```python
from build123d import *

# Parameters (mm, degrees)
ESTRUSIONE_ESTRUSIONE1_DEPTH = 4.1
SCHIZZO2_R                   = 1.25
TAGLIO_ESTRUSIONE1_DEPTH     = 4.1
RACCORDO1_DEPTH              = 4.1
RACCORDO2_R                  = 11


with BuildPart() as part:
    # Schizzo1 → Estrusione-Estrusione1 (new body)
    with BuildSketch(Plane.XY):
        with BuildLine():
            Line((-12, 0), (-12, 8))
            Line((-12, 8), (23.997894166, 8))
            Line((23.997894166, 8), (38.008621711, 8))
            Line((38.008621711, 8), (38.008621711, -12))
            Line((38.008621711, -12), (0, -12))
            ThreePointArc((0, -12), (-8.485281374, -8.485281374), (-12, 0))
        make_face()
    extrude(amount=ESTRUSIONE_ESTRUSIONE1_DEPTH)

    # Schizzo2 → Taglio-Estrusione1 (cut)
    with BuildSketch(Plane.XY.offset(4.1)):
        with Locations((-2, -2.1)):
            Circle(SCHIZZO2_R)
        with Locations((28, -2.1)):
            Circle(SCHIZZO2_R)
        with Locations((18, -2.1)):
            Circle(SCHIZZO2_R)
    extrude(amount=-TAGLIO_ESTRUSIONE1_DEPTH, mode=Mode.SUBTRACT)

    # Raccordo1: read off the stored shape, not the designer's step
    # Raccordo1 outline → Raccordo1 (cut)
    with BuildSketch(Plane.XY):
        with BuildLine():
            ThreePointArc((-12, 0), (-8.485281374, -8.485281374), (0, -12))
            ThreePointArc((0, -12), (-10, -2), (0, 8))
            Line((0, 8), (-12, 8))
            Line((-12, 8), (-12, 0))
        make_face()
    extrude(amount=RACCORDO1_DEPTH, mode=Mode.SUBTRACT)

    # Raccordo2
    raccordo2_edges = [part.edges().sort_by_distance(p)[0] for p in [
        (38.008621711, -12, 2.05),
    ]]
    fillet(raccordo2_edges, radius=RACCORDO2_R)


solid = part.part
```
The listing builds one solid part. Answer for the finished solid, in the listing's coordinates (mm). Give positions to 0.01 mm unless a question says otherwise; leave off trailing zeros. Write each loop counter-clockwise with the first axis right and the second up, starting at its lowest first coordinate (ties: lowest second). Pieces come first, ordered by that corner, then holes. Notation, with made-up numbers: M 55.5,3 L 110.5,3 A15 ccw 110.5,15 Z; hole C 86,80 d11. An arc over 180 degrees is marked long. Write each question's results on one line, items separated by ' | '.
Q1. Section C-C, the plane y = -2.1 is taken. Write down the section's boundary in (x, z).
Output values:
outline: M -10,0 L -3.25,0 L -3.25,4.1 L -10,4.1 Z; M -0.75,0 L 16.75,0 L 16.75,4.1 L -0.75,4.1 Z; M 19.25,0 L 26.75,0 L 26.75,4.1 L 19.25,4.1 Z; M 29.25,0 L 37.95,0 L 37.95,4.1 L 29.25,4.1 Z
Q2. A flat-ended cylindrical pin translates along its axis: P1, Ø2, axis at x = 28, y = -2.1, coming from the -Z side. Find the tip coordinate at first contact, or state that the pin passes through.
Output values:
P1: through
Q3. Consider L1, parallel to Y at x = 18, z = 3; L2, parallel to X at y = -1.75, z = 0.95; L3, parallel to X at y = -2.75, z = 0.35. Determine where each line is inside the solid, lowest interval first. Write a range as from..to.
Output values:
L1: -12..-3.35, -0.85..8 | L2: -10..-3.2, -0.8..16.8, 19.2..26.8, 29.2..37.98 | L3: -9.97..-3.07, -0.93..16.93, 19.07..26.93, 29.07..37.87
Q4. Section A-A, the plane x = 18 is taken. Write down the section's boundary in (y, z).
Output values:
outline: M -12,0 L -3.35,0 L -3.35,4.1 L -12,4.1 Z; M -0.85,0 L 8,0 L 8,4.1 L -0.85,4.1 Z
Q5. Section B-B, the plane z = 0.45 is taken. Write down the section's boundary in (x, y), then the cut area to 3 significant figures.
Output values:
outline: M 0,-12 L 27.01,-12 A11 ccw 38.01,-1 L 38.01,8 L 0,8 A10 ccw Z; hole C -2,-2.1 d2.5; hole C 18,-2.1 d2.5; hole C 28,-2.1 d2.5 | area: 877 mm2
Q6. Section D-D, the plane x = 28 is taken. Write down the section's boundary in (y, z).
Output values:
outline: M -11.96,0 L -3.35,0 L -3.35,4.1 L -11.96,4.1 Z; M -0.85,0 L 8,0 L 8,4.1 L -0.85,4.1 Z
Q7. For a pull along X with two mould halves and no side action, classify faces 1 (the flat face through (14, -2, 4.1)), 2 (the cylindrical face through (-10, -2, 2)), 3 (the cylindrical face through (-0.81, -1.72, 2.08)) as released by +X, released by -X, zero draft, split by the parting line, or undercut.
Output values:
face 1: zero draft | face 2: released by -X | face 3: undercut
